Study the drawing (mm; zero at the part's minimum x, y, z) and answer. A direction names the side the tool comes from. Round coordinates to 2 decimals unless told otherwise and drop trailing zeros. Order: outer loops, then holes, each group sorted by start corner. A loop starts at its lowest first (then second) coordinate and runs counter-clockwise, first axis right, second up. Notation, with made-up numbers: (47.5, 7) -> (106.5, 7) arc R27 cw to (106.5, 32) -> close; hole circle Ø10 at (-4.5, 36). An arc over 180 degrees is marked (long way). Use one line per item in the form item = value.
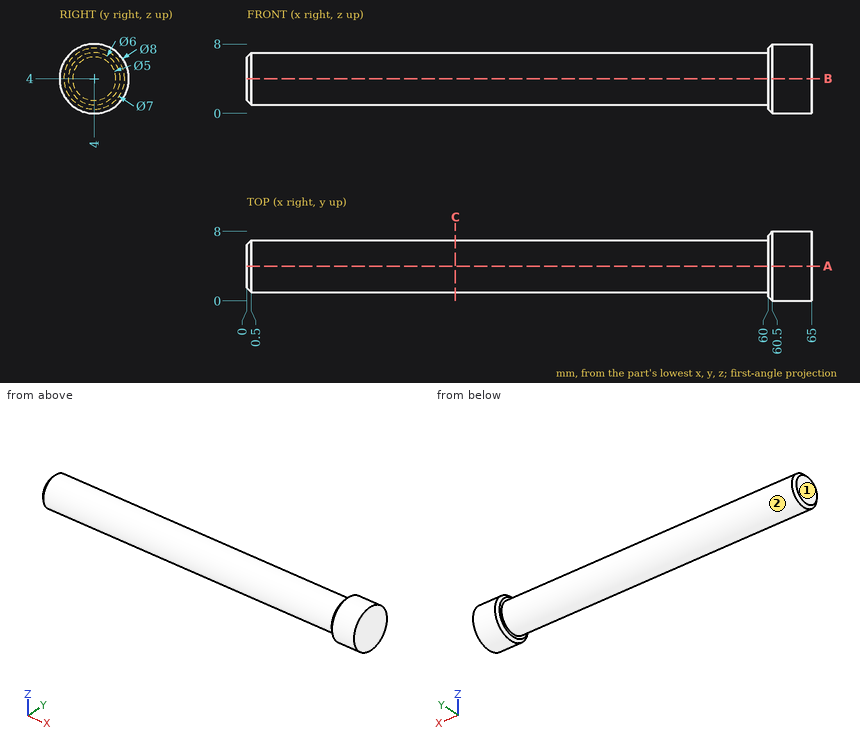
Item 1: The part is cut by section C-C, the plane x = 24. Give the vertices of the cut face in (y, z), and give its area (3 significant figures).
Findings:
outline = circle Ø6 at (4, 4)
area = 28.3 mm^2
Item 2: For the marked faces 1 and 2, determine the directions among +Z, -Z, +X, -X, +Y, -Y from which every point of the face is accessible in a straight line to the end or side of a thin tool.
Findings:
face_1 = +Z, -Z, -X, +Y, -Y
face_2 = -X
Item 3: The part is cut by section A-A, the plane y = 4. Give the vertices of the cut face in (x, z), and give its area (4 significant figures).
Findings:
outline = (0, 1.5) -> (0.5, 1) -> (60, 1) -> (60, 0.5) -> (60.5, 0) -> (65, 0) -> (65, 8) -> (60.5, 8) -> (60, 7.5) -> (60, 7) -> (0.5, 7) -> (0, 6.5) -> close
area = 399.5 mm^2
Item 4: Flat-ended cylindrical pins translate along their axes: P1, Ø1.5, axis at x = 9, z = 4, coming from the +Y side; P2, Ø2, axis at x = 28, z = 6.5, coming from the -Y side. Find the tip coordinate at first contact, or state that the pin passes through.
Findings:
P1 = 7
P2 = 1.4
Item 5: Consider line 1 along X through (y, z) = (5.75, 6.75); line 2 along Z through (x, y) = (45, 4.25); line 3 along X through (y, z) = (6, 6). Determine where each line is inside the solid, lowest interval first.
Findings:
line_1 = 60 to 65
line_2 = 1.01 to 6.99
line_3 = 0.33 to 65
